For this review, take the finished solid that the model builds, in its own axes (mm). A direction names the side the tool comes from. Coordinates: 2 decimals unless noted, no trailing zeros. Write each loop counter-clockwise with the first axis right and the second up, starting at its lowest first coordinate (ties: lowest second). Pieces come first, ordered by that corner, then holes.
1) We need section C-C on y = 12.25. Write out the cut boundary in (x, z), then the cut area to 3 significant figures.
2) We need section A-A on y = 1.75. Write out the cut boundary in (x, z), then the cut area to 3 significant figures.
3) For faces 5 (the face through (5.3, 18.5, 0)), 6 (the face through (0, 0, 0)), 7 (the face through (-0.9, 1.15, -2.86)), list the 3-axis set-ups (+Z, -Z, +X, -X, +Y, -Y) from which the entire face can be reached by the end or side of a thin tool; tool diameter is ignored.
4) Insertion check: P1, Ø2, axis at x = -4.5, z = 0, coming from the +Y side; P2, Ø12, axis at y = 15.5, z = -9, coming from the +X side; P3, Ø10, axis at x = 5.5, y = 8.5, coming from the +Z side; P4, Ø12, axis at y = 6, z = -5, coming from the +X side. Each pin has a flat end and moves straight along its axis. Give the tip position at first contact, or say it passes through.
5) To check wall thickness, follow line 1 along Y through (x, z) = (2, -3.5); line 2 along Y through (x, z) = (0, 1.5); line 3 along X through (y, z) = (4.95, -8). State the ranges of each line that lie inside material, in increasing order.
6) Mouldability with a two-part tool opening along Y and no side actions: class faces 1 (the face through (-4.61, 16.6, 0.08)), 2 (the face through (3.4, 5, 10.2)), 3 (the face through (0.17, 18.48, -3.72)), 4 (the face through (-0.075, 6.397, -8.117)) as pulls with the +Y half, pulls with the -Y half, needs draft (parallel to the pull), parting line crosses it, or undercut.
7) We need section B-B on y = 16. Write out the cut boundary in (x, z).
from build123d import *

# Parameters (mm, degrees)
M2_GEWINDEBOHRUNG1_D     = 1.6
M2_GEWINDEBOHRUNG1_DEPTH = 3
M2_GEWINDEBOHRUNG1_TIP   = 0.480688495
M2_GEWINDEBOHRUNG2_D     = 1.6
M2_GEWINDEBOHRUNG2_DEPTH = 5
M2_GEWINDEBOHRUNG2_TIP   = 0.480688495


with BuildPart() as part:
    # Skizze1 → Rotation1 (revolve)
    with BuildSketch(Plane.XY, mode=Mode.PRIVATE) as rotation1_sk:
        Polygon((9.5, 1), (3, 1), (3, 1.3), (1, 1.3), (1, 0), (0, 0), (0, 23.8), (1, 23.8), (1, 20), (8.5, 20), (11.5, 15), (11.5, 5.5), (10.5, 5.5), (10.5, 5), (11.5, 5), (11.5, 2.5), align=None)
    revolve(rotation1_sk.sketch.rotate(Axis((0, 0, 0), (0, 1, 0)), 90), axis=Axis((0, 0, 0), (0, 1, 0)))

    # M2 Gewindebohrung1
    with Locations(Plane(origin=(0, 20, 0), x_dir=(1, 0, 0), z_dir=(0, 1, 0))):
        with Locations((-4.5, 0), (0, 4.5), (4.5, 0), (0, -4.5)):
            Hole(M2_GEWINDEBOHRUNG1_D / 2, depth=M2_GEWINDEBOHRUNG1_DEPTH)
            with Locations((0, 0, -(M2_GEWINDEBOHRUNG1_DEPTH + M2_GEWINDEBOHRUNG1_TIP / 2))):  # 118° drill point
                Cone(0, M2_GEWINDEBOHRUNG1_D / 2, M2_GEWINDEBOHRUNG1_TIP, mode=Mode.SUBTRACT)

    # M2 Gewindebohrung2
    with Locations(Plane(origin=(0, 1, 0), x_dir=(-1, 0, 0), z_dir=(0, -1, 0))):
        with Locations((0, 8), (0, -8), (6, 0), (-6, 0)):
            Hole(M2_GEWINDEBOHRUNG2_D / 2, depth=M2_GEWINDEBOHRUNG2_DEPTH)
            with Locations((0, 0, -(M2_GEWINDEBOHRUNG2_DEPTH + M2_GEWINDEBOHRUNG2_TIP / 2))):  # 118° drill point
                Cone(0, M2_GEWINDEBOHRUNG2_D / 2, M2_GEWINDEBOHRUNG2_TIP, mode=Mode.SUBTRACT)


solid = part.part
Result:
1. outline: circle Ø23 at (0, 0)
1. area: 415 mm2
2. outline: circle Ø21 at (0, 0); hole circle Ø1.6 at (-6, 0); hole circle Ø1.6 at (0, -8); hole circle Ø1.6 at (0, 8); hole circle Ø1.6 at (6, 0)
2. area: 338 mm2
3. face 5: +Y
3. face 6: +Z, -Z, +X, -X, -Y
3. face 7: -Y
4. P1: stops at y = 20
4. P2: stops at x = 11.1
4. P3: stops at z = 11.49
4. P4: stops at x = 11.5
5. line 1: y = 1 to 20
5. line 2: y = 1.3 to 20
5. line 3: x = -8.26 to -0.8, 0.8 to 8.26
6. face 1: pulls with the +Y half
6. face 2: undercut
6. face 3: needs draft
6. face 4: pulls with the -Y half
7. outline: circle Ø21.8 at (0, 0)
